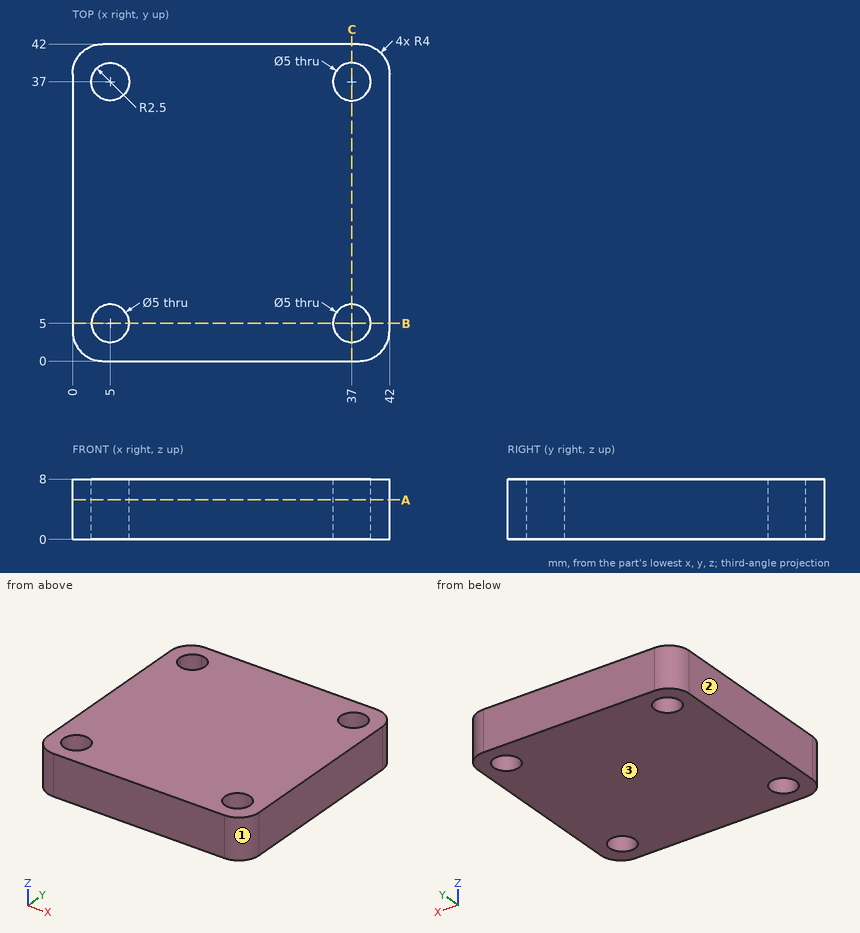
Geometry check sheet. Reference: drawing and pictorial views, mm from the part's lowest x, y, z. Give positions to 0.01 mm unless a question says otherwise; leave off trailing zeros. Order: outer loops, then holes, each group sorted by start corner. A loop starts at its lowest first (then second) coordinate and runs counter-clockwise, first axis right, second up. Notation, with made-up numbers: (-35, 20.25) -> (12, 20.25) arc R29 ccw to (12, 47.25) -> close; hole circle Ø9 at (25, 68). An arc over 180 degrees is marked (long way). Write each question's results on one line, items separated by ' | '. Start each with the question number.
(1) Gauge pin test, flat end, axial feed: P1, Ø4.5, axis at x = 37, y = 37, coming from the -Z side. Record the tip position at first contact, or that the pin passes through.
(2) Scan lines: line 1 (Y direction, x = 37, z = 3); line 2 (X direction, y = 7, z = 5.25); line 3 (Y direction, x = 3, z = 5.25). Record each from-to range of solid material in increasing order.
(3) Sectioned sample at B-B (y = 5). Enter the section's corners in (x, z), plus the area to 3 significant figures.
(4) Mould release check, pull along X, two halves, no side actions. Record for the marked faces 1, 2 and 3: pulls with the +X half, pulls with the -X half, needs draft (parallel to the pull), parting line crosses it, or undercut.
(5) Sectioned sample at A-A (z = 5.25). Enter the section's corners in (x, y).
Answer below:
1) P1: through
2) line 1: 0 to 2.5, 7.5 to 34.5, 39.5 to 42 | line 2: 0 to 3.5, 6.5 to 35.5, 38.5 to 42 | line 3: 0.13 to 3.5, 6.5 to 35.5, 38.5 to 41.87
3) outline: (0, 0) -> (2.5, 0) -> (2.5, 8) -> (0, 8) -> close; (7.5, 0) -> (34.5, 0) -> (34.5, 8) -> (7.5, 8) -> close; (39.5, 0) -> (42, 0) -> (42, 8) -> (39.5, 8) -> close | area: 256 mm2
4) face 1: pulls with the +X half | face 2: pulls with the -X half | face 3: needs draft
5) outline: (0, 4) arc R4 ccw to (4, 0) -> (38, 0) arc R4 ccw to (42, 4) -> (42, 38) arc R4 ccw to (38, 42) -> (4, 42) arc R4 ccw to (0, 38) -> close; hole circle Ø5 at (5, 5); hole circle Ø5 at (5, 37); hole circle Ø5 at (37, 5); hole circle Ø5 at (37, 37)
